Input: dimensioned drawing with shaded views. Units: mm. Origin: part minimum x, y, z. Give positions to 0.01 mm unless a question says otherwise; leave off trailing zeros. Order: outer loops, then holes, each group sorted by start corner. A loop starts at its lowest first (then second) coordinate and runs counter-clockwise, first axis right, second up.
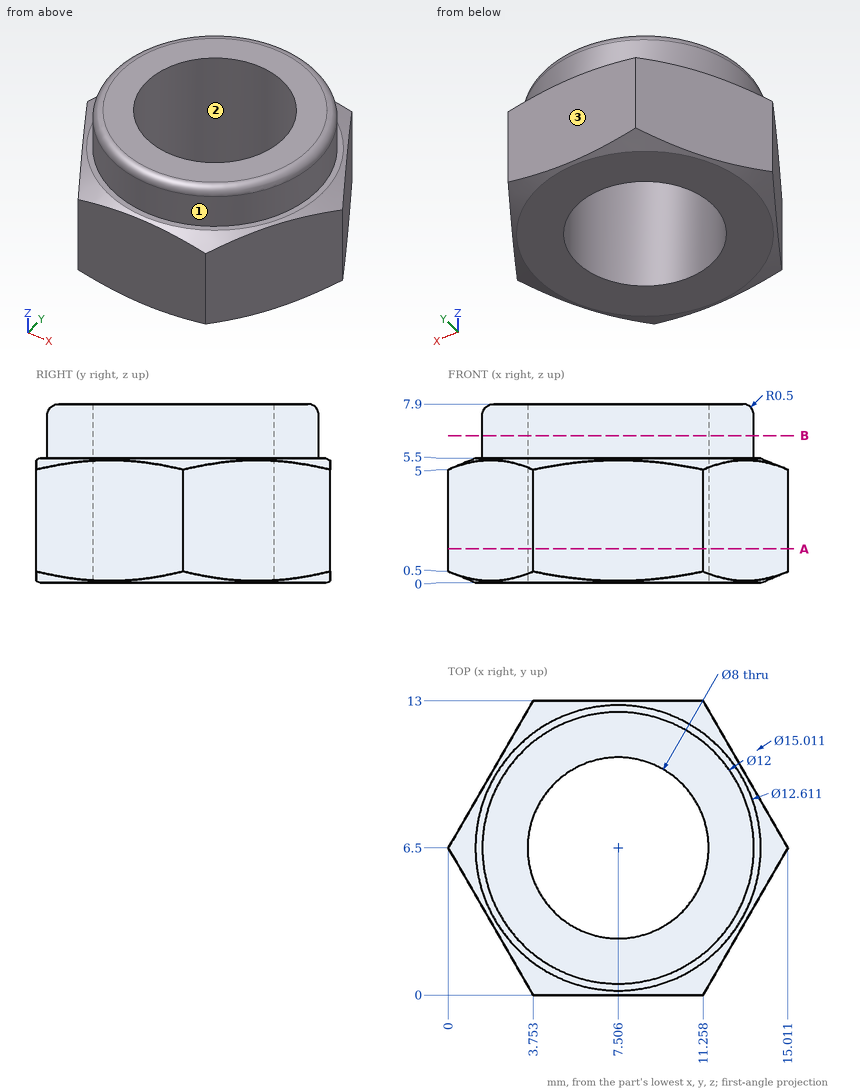
1) Material intervals for L1, parallel to Y at x = 7.5, z = 1.25; L2, parallel to X at y = 4.5, z = 2.5 (1 decimal); L3, parallel to X at y = 7, z = 4 (1 decimal), sorted ascending.
Report:
L1: y = 0 to 2.5, 10.5 to 13
L2: x = 1.2 to 4, 11 to 13.9
L3: x = 0.3 to 3.5, 11.5 to 14.7
2) Pin query (flat end, axial travel): pin 1 (3 mm diameter, centred on y = 9.5, z = 6.5, fed in from +X); pin 2 (1.5 mm diameter, centred on x = 1.5, z = 4, fed in from -Y) (1 decimal). Return the tip coordinate at first contact, or that it passes through.
Report:
pin 1: stops at x = 13.84
pin 2: stops at y = 2.6
3) Draft query along X for the marked faces 1, 2 and 3. Return one class per face: +X half, -X half, draft (parallel to the pull), parting line (faces both ways), or undercut.
Report:
face 1: parting line
face 2: undercut
face 3: draft
4) Section query A-A, the plane z = 1.5. Return the cut outline in (x, y) (1 decimal).
Report:
outline: (0, 6.5) - (3.8, 0) - (11.3, 0) - (15, 6.5) - (11.3, 13) - (3.8, 13) - close; hole circle Ø8 at (7.5, 6.5)
5) Section query B-B, the plane z = 6.5. Return the cut outline in (x, y) (1 decimal).
Report:
outline: circle Ø12 at (7.5, 6.5); hole circle Ø8 at (7.5, 6.5)
